Geometry check sheet. Reference: the model listing, model coordinates, mm. A direction names the side the tool comes from. Give positions to 0.01 mm unless a question says otherwise; leave off trailing zeros. Loops run counter-clockwise (first coordinate to the right, second up) from the corner with the lowest first, then second, coordinate; pieces in that order, holes last. Notation, with made-up numbers: (39, 81.25) - (48, 81.25) arc R25 ccw to (48, 118.25) - close; hole circle Ø7 at (41, 4.25). An arc over 180 degrees is marked (long way). One line per question, with ' | ' between items. Start each with the question number.
from build123d import *

# Parameters (mm, degrees)
SKETCH1_R           = 2.5
BOSS_EXTRUDE1_DEPTH = 17.5
CUT_EXTRUDE1_START  = -2
SKETCH3_W           = 5.788329994
SKETCH3_H           = 11.481307843
CUT_EXTRUDE1_DEPTH  = 35
CHAMFER1_SIZE       = 0.5


with BuildPart() as part:
    # Sketch1 → Boss-Extrude1 (new, symmetric)
    with BuildSketch(Plane(origin=(0, 0, 0), x_dir=(1, 0, 0), z_dir=(0, 1, 0))):
        with Locations(Location((0, 0, 0), (0, 0, 270))):
            Circle(SKETCH1_R)
    extrude(amount=BOSS_EXTRUDE1_DEPTH, both=True)

    # Sketch3 → Cut-Extrude1 (cut)
    with BuildSketch(Plane.XY.offset(CUT_EXTRUDE1_START)):
        with Locations((0, 13.740653921)):
            Rectangle(SKETCH3_W, SKETCH3_H)
        with Locations((0, -13.740653921)):
            Rectangle(SKETCH3_W, SKETCH3_H)
    extrude(amount=-CUT_EXTRUDE1_DEPTH, mode=Mode.SUBTRACT)

    # Chamfer1
    chamfer1_edges = [part.edges().sort_by_distance(p)[0] for p in [
        (-2.371708245, -17.5, 0.790569415),
        (0, -17.5, -2),
        (-2.371708245, 17.5, 0.790569415),
        (0, 17.5, -2),
    ]]
    chamfer(chamfer1_edges, length=CHAMFER1_SIZE - 0.0001)  # a hair under: the kernel refuses the full size


solid = part.part
(1) Section check B-B, the plane y = 5.5. Record the boundary of the cut face in (x, z).
(2) Tool access check on faces 1 (the face through (0, 13, -2)), 2 (the face through (0, -12, -2)), 3 (the face through (-0.075, 17.365, 2.134)). Record the directions out of +Z, -Z, +X, -X, +Y, -Y that give a thin tool (end or side, any length) a straight path to the whole face; none if there is none.
(3) Section check A-A, the plane x = 0. Record the boundary of the cut face in (y, z).
(4) Depth check by flat-ended pin: pin 1 Ø2 at (x, z) = (1, 2) entering from +Y; pin 2 Ø2 at (x, y) = (1, 13) entering from -Z. Enter the tip coordinate at first touch or a pass-through.
(5) Section check C-C, the plane y = -14.5. Record the boundary of the cut face in (x, z).
(6) Material ranges on line 1 (Y direction, x = -0.7, z = -2.1); line 2 (X direction, y = 6, z = 0.15); line 3 (X direction, y = 8, z = 0.75), recorded low to high.
Numbers:
1) outline: circle Ø5 at (0, 0)
2) face 1: -Z, +X, -X, +Y | face 2: -Z, +X, -X, -Y | face 3: +Y
3) outline: (-17.5, -1.5) - (-17, -2) - (-8, -2) - (-8, -2.5) - (8, -2.5) - (8, -2) - (17, -2) - (17.5, -1.5) - (17.5, 2) - (17, 2.5) - (-17, 2.5) - (-17.5, 2) - close
4) pin 1: y = 17.5 | pin 2: z = -2
5) outline: (-1.5, -2) - (1.5, -2) arc R2.5 ccw (long way) to start
6) line 1: -8 to 8 | line 2: -2.5 to 2.5 | line 3: -2.38 to 2.38
